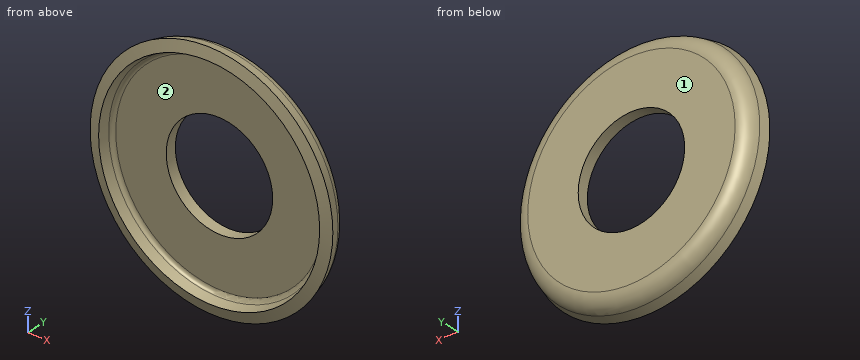
Autodesk Inventor part; units mm, degrees
ref_plane "YZ Plane" through (0, 0, 0) normal (1, 0, 0) x (0, 1, 0)
ref_plane "XZ Plane" through (0, 0, 0) normal (0, 1, 0) x (-1, 0, 0)
ref_plane "XY Plane" through (0, 0, 0) normal (0, 0, 1) x (1, 0, 0)
sketch "Schizzo1" plane through (0, 0, 0) normal (0, 0, 1) x (1, 0, 0)
  line L0 (4.75, 6.5534) -> (9.25, 6.5534)
  arc A0 (10.6023, 5.5157) -> (9.25, 6.5534) centre (9.25, 5.1534) ccw
  line L1 (4.75, 5.5534) -> (9.25, 5.5534)
  line L2 (4.75, 5.5534) -> (4.75, 6.5534)
  line L3 (0, 6.5534) -> (0, 3.993) construction
  arc A1 (9.6364, 5.2569) -> (9.25, 5.5534) centre (9.25, 5.1534) ccw
  line L4 (9.8599, 4.4226) -> (10.8258, 4.6814)
  line L5 (10.6023, 5.5157) -> (10.8258, 4.6814)
  line L6 (9.8599, 4.4226) -> (9.6364, 5.2569)
  point P0 (0, 0)
  dimension "d1" = 4.5
  dimension "d2" = 1
  dimension "d8" = 4.75
  dimension "d10" = 0.4
  dimension "d11" = 9.25
revolve "Rivoluzione1" add sketch "Schizzo1" angle 360 about axis through (0, 6.5534, 0) along (0, -1, 0)
properties part number "Rondella superiore"
Geometry: final body of the model. Coordinates: model frame, mm. Face numbers are marked on the shaded views. Coordinates: 2 decimals unless noted, no trailing zeros. Write each loop counter-clockwise with the first axis right and the second up, starting at its lowest first coordinate (ties: lowest second). Pieces come first, ordered by that corner, then holes. Notation, with made-up numbers: (-32.5, -31.75) - (-2.5, -31.75) arc R28 ccw to (-2.5, 4.25) - close; hole circle Ø5 at (-14.5, 2). An arc over 180 degrees is marked (long way). Return JSON: item names as keys, results as strings.
Item 1: Pin query (flat end, axial travel): pin 1 Ø9 at (x, z) = (-3, 3.5) entering from -Y. Return the tip coordinate at first contact, or that it passes through.
Completed:
{"pin 1": "stops at y = 5.55"}
Item 2: Line query: L1, parallel to Y at x = -1, z = 5.5; L2, parallel to X at y = 5.45, z = -2.75; L3, parallel to Z at x = 1, y = 6.2. Output: solid intervals per line, ascending.
Completed:
{"L1": "y = 5.55 to 6.55", "L2": "x = -10.26 to -9.11, 9.11 to 10.26", "L3": "z = -10.13 to -4.64, 4.64 to 10.13"}
Item 3: Section query A-A (z = 0). Output: boundary loops of the cut face in (x, y), and give its area (3 significant figures).
Completed:
{"outline": "(-10.83, 4.68) - (-9.86, 4.42) - (-9.64, 5.26) arc R0.4 cw to (-9.25, 5.55) - (-4.75, 5.55) - (-4.75, 6.55) - (-9.25, 6.55) arc R1.4 ccw to (-10.6, 5.52) - close; (4.75, 5.55) - (9.25, 5.55) arc R0.4 cw to (9.64, 5.26) - (9.86, 4.42) - (10.83, 4.68) - (10.6, 5.52) arc R1.4 ccw to (9.25, 6.55) - (4.75, 6.55) - close", "area": "13.1 mm2"}
Item 4: Section query C-C (y = 5.95). Output: boundary loops of the cut face in (x, z).
Completed:
{"outline": "circle Ø20.8 at (0, 0); hole circle Ø9.5 at (0, 0)"}
Item 5: Pull-direction query (X, two-part tool) for the marked faces 1 and 2; classes: +X half, -X half, draft (parallel to the pull), parting line (faces both ways), or undercut.
Completed:
{"face 1": "draft", "face 2": "undercut"}
Item 6: Section query B-B (x = 0). Output: boundary loops of the cut face in (y, z).
Completed:
{"outline": "(4.42, -9.86) - (4.68, -10.83) - (5.52, -10.6) arc R1.4 ccw to (6.55, -9.25) - (6.55, -4.75) - (5.55, -4.75) - (5.55, -9.25) arc R0.4 cw to (5.26, -9.64) - close; (4.42, 9.86) - (5.26, 9.64) arc R0.4 cw to (5.55, 9.25) - (5.55, 4.75) - (6.55, 4.75) - (6.55, 9.25) arc R1.4 ccw to (5.52, 10.6) - (4.68, 10.83) - close"}
